Source: CAD feature listing. Evaluate the final solid. Frame: model axes, mm. Give positions to 0.01 mm unless a question says otherwise; leave off trailing zeros. Order: outer loops, then holes, each group sorted by start corner. A loop starts at its lowest first (then second) coordinate and runs counter-clockwise, first axis right, second up. Notation, with made-up numbers: M 48.25,86.25 L 74.25,86.25 A10 ccw 74.25,95.25 Z; hole C 52,-5 d8. An arc over 180 degrees is marked long. Answer in a Markdown table with one row per item. Add a question column.
(1) Section query A-A, the plane x = -12.5. Return loops of the section in (y, z), plus the area to 3 significant figures.
(2) Pin query (flat end, axial travel): P1, Ø3.5, axis at x = -7.5, y = 120, coming from the +Z side; P2, Ø4, axis at y = 81.5, z = -254.5, coming from the +X side; P3, Ø6, axis at y = 30, z = -495, coming from the +X side. Return the tip coordinate at first contact, or that it passes through.
(3) Section query B-B, the plane z = -259.5. Return loops of the section in (x, y), plus the area to 4 significant figures.
(4) Material intervals for line 1 along Y through (x, z) = (-7.5, -2); line 2 along Y through (x, z) = (-4, -373); line 3 along Y through (x, z) = (-7.5, -495), sorted ascending.
from build123d import *

# Parameters (mm, degrees)
SKETCH2_W                                         = 500
SKETCH2_H                                         = 150
BASE_EXTRUDE_DEPTH                                = 15
SKETCH3_W                                         = 10
SKETCH3_H                                         = 14
CUT_EXTRUDE1_DEPTH                                = 523.230791892
SKETCH4_W                                         = 5
SKETCH4_H                                         = 5
CUT_EXTRUDE2_DEPTH                                = 523.230791892
CSK_FOR_M3_5_FLAT_HEAD_MACHINE_SCREW1_D           = 3.9
CSK_FOR_M3_5_FLAT_HEAD_MACHINE_SCREW1_CSINK_D     = 8.2
CSK_FOR_M3_5_FLAT_HEAD_MACHINE_SCREW1_CSINK_ANGLE = 90
M3_0_3_000000_DIAMETER_HOLE1_D                    = 3
M3_0_3_000000_DIAMETER_HOLE1_DEPTH                = 10
M3_0_3_000000_DIAMETER_HOLE1_TIP                  = 0.901290929


with BuildPart() as part:
    # Sketch2 → Base-Extrude (new body)
    with BuildSketch(Plane(origin=(0, 0, 0), x_dir=(0, 0, -1), z_dir=(1, 0, 0))):
        with Locations((250, 75)):
            Rectangle(SKETCH2_W, SKETCH2_H)
    extrude(amount=-BASE_EXTRUDE_DEPTH)

    # Sketch3 → Cut-Extrude1 (cut, through all)
    with BuildSketch(Plane.XY):
        with Locations((-5, 77)):
            Rectangle(SKETCH3_W, SKETCH3_H)
    extrude(amount=-CUT_EXTRUDE1_DEPTH, mode=Mode.SUBTRACT)

    # Sketch4 → Cut-Extrude2 (cut, through all)
    with BuildSketch(Plane.XY):
        with Locations((-12.5, 12.5)):
            Rectangle(SKETCH4_W, SKETCH4_H)
    extrude(amount=-CUT_EXTRUDE2_DEPTH, mode=Mode.SUBTRACT)

    # CSK for M3.5 Flat Head Machine Screw1 (through all)
    with Locations(Plane(origin=(0, 0, 0), x_dir=(0, 0, -1), z_dir=(1, 0, 0))):
        with Locations((495, 140), (495, 30)):
            CounterSinkHole(CSK_FOR_M3_5_FLAT_HEAD_MACHINE_SCREW1_D / 2, CSK_FOR_M3_5_FLAT_HEAD_MACHINE_SCREW1_CSINK_D / 2, counter_sink_angle=CSK_FOR_M3_5_FLAT_HEAD_MACHINE_SCREW1_CSINK_ANGLE)

    # M3.0 (3.000000) Diameter Hole1
    with Locations(Plane.XY):
        with Locations((-7.5, 30), (-7.5, 120)):
            Hole(M3_0_3_000000_DIAMETER_HOLE1_D / 2, depth=M3_0_3_000000_DIAMETER_HOLE1_DEPTH)
            with Locations((0, 0, -(M3_0_3_000000_DIAMETER_HOLE1_DEPTH + M3_0_3_000000_DIAMETER_HOLE1_TIP / 2))):  # 118° drill point
                Cone(0, M3_0_3_000000_DIAMETER_HOLE1_D / 2, M3_0_3_000000_DIAMETER_HOLE1_TIP, mode=Mode.SUBTRACT)


solid = part.part
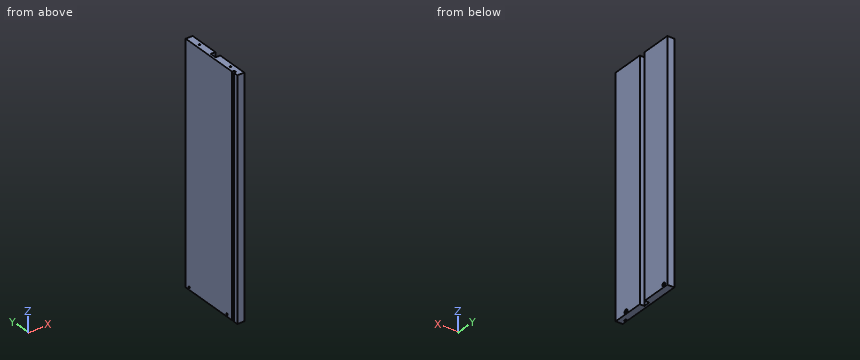
Values follow:
| question | item | result |
|---|---|---|
| 1 | outline | M 0,-500 L 10,-500 L 10,0 L 0,0 Z; M 15,-500 L 150,-500 L 150,0 L 15,0 Z; hole C 30,-495 d3.9; hole C 140,-495 d3.9 |
| 1 | area | 72,500 mm² |
| 2 | P1 | stops at z = 0 |
| 2 | P2 | stops at x = -10 |
| 2 | P3 | stops at x = -1.1 |
| 3 | outline | M -15,0 L 0,0 L 0,70 L -10,70 L -10,84 L 0,84 L 0,150 L -15,150 L -15,15 L -10,15 L -10,10 L -15,10 Z |
| 3 | area | 2,085 mm² |
| 4 | line 1 | y = 0 to 28.5, 31.5 to 70, 84 to 118.5, 121.5 to 150 |
| 4 | line 2 | y = 0 to 70, 84 to 150 |
| 4 | line 3 | y = 0 to 28.05, 31.95 to 70, 84 to 138.05, 141.95 to 150 |
